from build123d import *

# Parameters (mm, degrees)
CHAMFER_2_SIZE = 0.4


with BuildPart() as part:
    # Эскиз1 → Повернуть1 (revolve)
    with BuildSketch(Plane.XY, mode=Mode.PRIVATE) as revolve_1_sk:
        Polygon((-6.35, 25), (-6.35, 10), (-2.5, 10), (-2.5, 9), (-1.85, 9), (-1.85, 0), (0, 0), (0, 11.499600798), (-2, 11.499600798), (-2, 25), (-3.85, 25), (-3.85, 11.499600798), (-4.5, 11.499600798), (-4.5, 25), align=None)
    revolve(revolve_1_sk.sketch.rotate(Axis((0, 11.499600798, 0), (0, -1, 0)), 270), axis=Axis((0, 11.499600798, 0), (0, -1, 0)))

    # Фаска2
    chamfer_2_edges = [part.edges().sort_by_distance(p)[0] for p in [
        (0, 0, -1.85),
        (0, 10, -6.35),
        (0, 25, -6.35),
        (0, 25, -4.5),
        (0, 25, -3.85),
        (0, 25, -2),
    ]]
    chamfer(chamfer_2_edges, length=CHAMFER_2_SIZE)


solid = part.part
CAD build for the part. Positions are in the model's coordinates, mm. A direction names the side the tool comes from. Give positions to 0.01 mm unless a question says otherwise; leave off trailing zeros. Loops run counter-clockwise (first coordinate to the right, second up) from the corner with the lowest first, then second, coordinate; pieces in that order, holes last. Notation, with made-up numbers: M -4.75,-23.5 L 8.25,-23.5 A20 ccw 8.25,-18.5 Z; hole C 46.5,76.5 d5. An arc over 180 degrees is marked long. One line per question, with ' | ' between items. Start each with the question number.
1. Two-plate mould, pull along Z, no slides. Class faces 4 (the face through (3.86, 17.4, -5.04)), 5 (the face through (-1.352, 18.142, 4.292)), 6 (the face through (2.3, 25, -1.5)): pulls with the +Z half, pulls with the -Z half, needs draft (parallel to the pull), parting line crosses it, or undercut.
2. 3-axis set-ups, long thin cutter, end or side, ignore diameter. For faces 1 (the face through (0, 0, 0)), 2 (the face through (1.806, 4.64, -0.401)), 3 (the face through (2, 18, 0)): which of +Z, -Z, +X, -X, +Y, -Y reach the whole face in a straight line?
3. Flat gauge pins, fed straight in: pin 1 (2 mm diameter, centred on y = 5, z = 2, fed in from +X); pin 2 (3 mm diameter, centred on x = 0.5, z = 0.5, fed in from +Y); pin 3 (2.5 mm diameter, centred on x = 0, z = 0, fed in from +Y); pin 4 (1.5 mm diameter, centred on y = 8.5, z = -4, fed in from +X). Where does each tip first touch, or does it go through?
4. Saw through at A-A on y = 20.5. Give the cut face in (x, z), plus the area to 3 significant figures.
5. Probe L1, parallel to X at y = 18, z = 0; L2, parallel to Z at x = -2.5, y = 14; L3, parallel to X at y = 23, z = -1.25. List the from-to ranges inside material, lowest first. Write a range as from..to.
6. Saw through at B-B on y = 8. Give the cut face in (x, z).
Result sheet:
1) face 4: parting line crosses it | face 5: undercut | face 6: needs draft
2) face 1: +Z, -Z, +X, -X, -Y | face 2: -Y | face 3: +Y
3) pin 1: stops at x = 1.56 | pin 2: stops at y = 24.81 | pin 3: stops at y = 11.5 | pin 4: passes through
4) outline: C 0,0 d12.7; C 0,0 d7.7; hole C 0,0 d9; hole C 0,0 d4 | area: 97.1 mm^2
5) L1: x = -6.35..-4.5, -3.85..-2, 2..3.85, 4.5..6.35 | L2: z = -5.84..-3.74, -2.93..2.93, 3.74..5.84 | L3: x = -6.23..-4.32, -3.64..-1.56, 1.56..3.64, 4.32..6.23
6) outline: C 0,0 d3.7
